Check sheet for the drawn part. Datum: minimum x, y, z corner. Units: mm. A direction names the side the tool comes from. Round coordinates to 2 decimals unless told otherwise and drop trailing zeros. Write each loop counter-clockwise with the first axis right and the second up, starting at its lowest first coordinate (ties: lowest second). Pieces come first, ordered by that corner, then holes.
Item 1: Cross-section at A-A on x = 37.5. Enter the section's corners in (y, z) (3 decimals), plus the area to 3 significant figures.
Item 2: Cross-section at B-B on z = 69. Enter the section's corners in (x, y) (3 decimals).
Item 3: Go/stop test with flat-tipped pins: pin 1 Ø4 at (x, y) = (98.5, 39.5) entering from -Z (3 decimals); pin 2 Ø20.5 at (y, z) = (13, 44) entering from +X; pin 3 Ø3.5 at (x, z) = (178, 81) entering from -Y. Record where each tip stops, or that it passes through.
Item 4: Tool access check on the marked faces 1 and 2. Record the directions out of +Z, -Z, +X, -X, +Y, -Y that give a thin tool (end or side, any length) a straight path to the whole face; none if there is none.
Item 5: Material ranges on line 1 (Y direction, x = 6, z = 81) (3 decimals); line 2 (Y direction, x = 177.8, z = 80.45) (3 decimals); line 3 (Z direction, x = 124, y = 40) (3 decimals), recorded low to high.
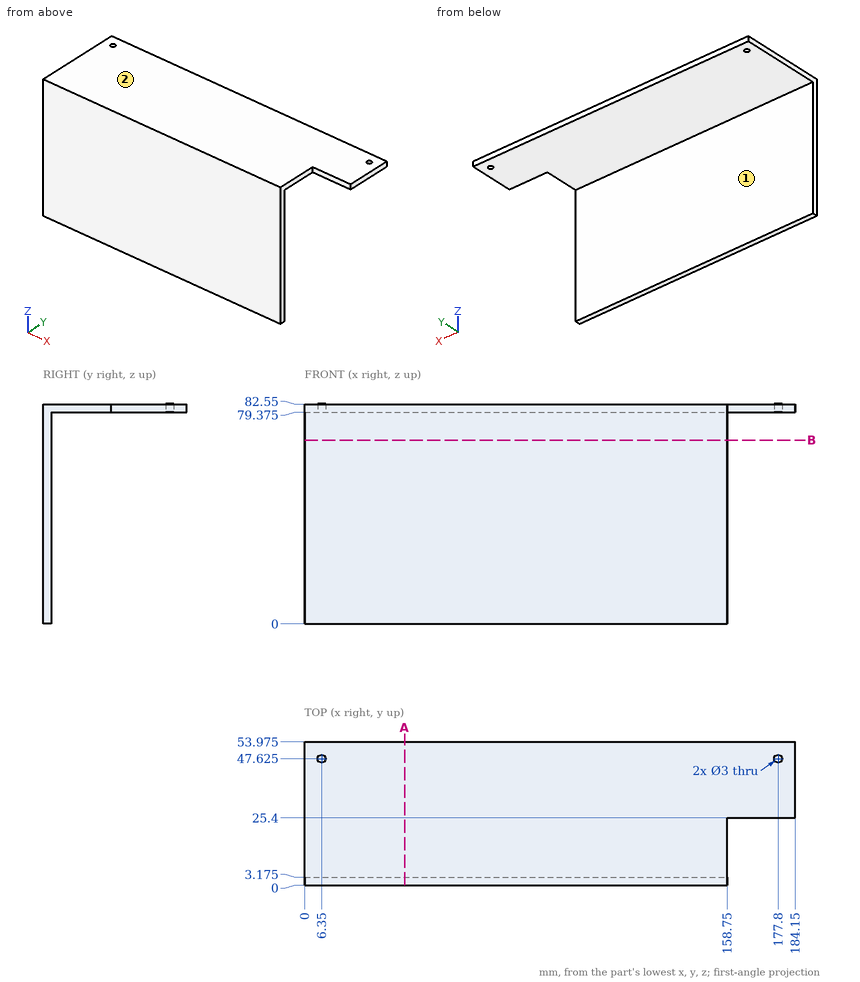
Response values:
1. outline: (0, 0) - (3.175, 0) - (3.175, 79.375) - (53.975, 79.375) - (53.975, 82.55) - (0, 82.55) - close
1. area: 423 mm2
2. outline: (0, 0) - (158.75, 0) - (158.75, 3.175) - (0, 3.175) - close
3. pin 1: stops at z = 79.375
3. pin 2: stops at x = 158.75
3. pin 3: stops at y = 25.4
4. face 1: -Z, +X, -X, +Y
4. face 2: +Z, +X, -X, +Y, -Y
5. line 1: y = 0 to 46.166, 49.084 to 53.975
5. line 2: y = 25.4 to 46.125, 49.125 to 53.975
5. line 3: z = 79.375 to 82.55
